from build123d import *

# Parameters (mm, degrees)
SKETCH1_W           = 120
SKETCH1_H           = 125
BOSS_EXTRUDE1_DEPTH = 70
SKETCH3_W           = 47
SKETCH3_H           = 9.5
CUT_EXTRUDE1_DEPTH  = 47
SKETCH4_W           = 43
SKETCH4_H           = 15
CUT_EXTRUDE2_DEPTH  = 47
CUT_REVOLVE1_ANGLE  = 120
SKETCH9_W           = 20
SKETCH9_H           = 47
CUT_EXTRUDE3_DEPTH  = 3
SKETCH10_W          = 20
SKETCH10_H          = 1.6
CUT_EXTRUDE4_DEPTH  = 3.5
CUT_EXTRUDE5_DEPTH  = 1
SKETCH13_W          = 71.5
SKETCH13_H          = 22.8
CUT_EXTRUDE6_DEPTH  = 5
SKETCH14_R          = 5
CUT_EXTRUDE7_DEPTH  = 10
SKETCH15_R          = 8
CUT_EXTRUDE8_DEPTH  = 1
SKETCH16_W          = 70
SKETCH16_H          = 18
CUT_EXTRUDE9_DEPTH  = 10
SKETCH17_W          = 70
SKETCH17_H          = 9
SKETCH18_W          = 70
SKETCH18_H          = 9
SKETCH19_W          = 60
SKETCH19_H          = 15
CUT_EXTRUDE10_DEPTH = 60
CUT_REVOLVE4_ANGLE  = 90
SKETCH21_W          = 120
SKETCH21_H          = 125
CUT_EXTRUDE11_DEPTH = 20
FILLET1_R           = 3
FILLET2_R           = 3
SKETCH22_W          = 11.5
SKETCH22_H          = 18.1
CUT_EXTRUDE12_DEPTH = 7


# Some blends are built 0.0001 mm under size
with BuildPart() as part:
    # Sketch1 → Boss-Extrude1 (new body)
    with BuildSketch(Plane(origin=(0, 0, 0), x_dir=(1, 0, 0), z_dir=(0, 1, 0))):
        with Locations((60, 62.5)):
            Rectangle(SKETCH1_W, SKETCH1_H)
    extrude(amount=BOSS_EXTRUDE1_DEPTH)

    # Sketch3 → Cut-Extrude1 (cut)
    with BuildSketch(Plane.XY):
        with Locations((26.5, 50.25)):
            Rectangle(SKETCH3_W, SKETCH3_H)
    extrude(amount=-CUT_EXTRUDE1_DEPTH, mode=Mode.SUBTRACT)

    # Sketch4 → Cut-Extrude2 (cut)
    with BuildSketch(Plane.XY):
        with Locations((26.5, 62.5)):
            Rectangle(SKETCH4_W, SKETCH4_H)
    extrude(amount=-CUT_EXTRUDE2_DEPTH, mode=Mode.SUBTRACT)

    # Cut-Sweep1: sweep along a path in Sketch5
    with BuildLine(Plane.XY) as cut_sweep1_path:
        Line((9, 45.5), (9, 33))
        ThreePointArc((9, 33), (10.464466094, 29.464466094), (14, 28))
        Line((14, 28), (39, 28))
        ThreePointArc((39, 28), (42.535533906, 29.464466094), (44, 33))
        Line((44, 33), (44, 45.5))
    # Sketch6 → Cut-Sweep1 (sweep, cut)
    with BuildSketch(Plane(origin=(0, 45.5, 0), x_dir=(1, 0, 0), z_dir=(0, 1, 0))):
        with BuildLine():
            Line((7, 0), (7, 2))
            ThreePointArc((7, 2), (9, 4), (11, 2))
            Line((11, 2), (11, 0))
            Line((11, 0), (7, 0))
        make_face()
    sweep(path=cut_sweep1_path.line, mode=Mode.SUBTRACT)

    # Sketch7 → Cut-Revolve1 (revolve, cut)
    with BuildSketch(Plane.XY):
        with BuildLine():
            Line((19.5, 30), (33.5, 30))
            ThreePointArc((33.5, 30), (26.5, 37), (19.5, 30))
        make_face()
    revolve(axis=Axis((19.5, 30, 0), (-1, 0, 0)), revolution_arc=CUT_REVOLVE1_ANGLE, mode=Mode.SUBTRACT)

    # Sketch9 → Cut-Extrude3 (cut)
    with BuildSketch(Plane(origin=(0, 45.5, 0), x_dir=(1, 0, 0), z_dir=(0, 1, 0))):
        with Locations((26.5, 23.5)):
            Rectangle(SKETCH9_W, SKETCH9_H)
    extrude(amount=-CUT_EXTRUDE3_DEPTH, mode=Mode.SUBTRACT)

    # Sketch10 → Cut-Extrude4 (cut)
    with BuildSketch(Plane.XY.offset(-47)):
        with Locations((26.5, 47.5)):
            Rectangle(SKETCH10_W, SKETCH10_H)
    extrude(amount=-CUT_EXTRUDE4_DEPTH, mode=Mode.SUBTRACT)

    # Sketch11 → Cut-Extrude5 (cut)
    with BuildSketch(Plane(origin=(0, 70, 0), x_dir=(1, 0, 0), z_dir=(0, 1, 0))):
        with BuildLine():
            Line((54.58, 81.89), (113.38, 81.89))
            ThreePointArc((113.38, 81.89), (116.972102448, 80.402102448), (118.46, 76.81))
            Line((118.46, 76.81), (118.46, 10.08))
            ThreePointArc((118.46, 10.08), (116.972102448, 6.487897552), (113.38, 5))
            Line((113.38, 5), (54.58, 5))
            ThreePointArc((54.58, 5), (50.987897552, 6.487897552), (49.5, 10.08))
            Line((49.5, 10.08), (49.5, 76.81))
            ThreePointArc((49.5, 76.81), (50.987897552, 80.402102448), (54.58, 81.89))
        make_face()
    extrude(amount=-CUT_EXTRUDE5_DEPTH, mode=Mode.SUBTRACT)

    # Sketch13 → Cut-Extrude6 (cut)
    with BuildSketch(Plane(origin=(0, 70, 0), x_dir=(1, 0, 0), z_dir=(0, 1, 0))):
        with Locations((64.25, 101.6)):
            Rectangle(SKETCH13_W, SKETCH13_H)
    extrude(amount=-CUT_EXTRUDE6_DEPTH, mode=Mode.SUBTRACT)

    # Sketch14 → Cut-Extrude7 (cut)
    with BuildSketch(Plane(origin=(0, 70, 0), x_dir=(1, 0, 0), z_dir=(0, 1, 0))):
        with Locations(Location((25, 67, 0), (0, 0, 270))):
            Circle(SKETCH14_R)
    extrude(amount=-CUT_EXTRUDE7_DEPTH, mode=Mode.SUBTRACT)

    # Sketch15 → Cut-Extrude8 (cut)
    with BuildSketch(Plane(origin=(0, 70, 0), x_dir=(1, 0, 0), z_dir=(0, 1, 0))):
        with Locations(Location((25, 67, 0), (0, 0, 270))):
            Circle(SKETCH15_R)
    extrude(amount=-CUT_EXTRUDE8_DEPTH, mode=Mode.SUBTRACT)

    # Sketch16 → Cut-Extrude9 (cut)
    with BuildSketch(Plane(origin=(120, 0, 0), x_dir=(0, 0, -1), z_dir=(1, 0, 0))):
        with Locations((80, 56)):
            Rectangle(SKETCH16_W, SKETCH16_H)
        with Locations((80, 36)):
            Rectangle(SKETCH16_W, SKETCH16_H)
    extrude(amount=-CUT_EXTRUDE9_DEPTH, mode=Mode.SUBTRACT)

    # Sketch17 → Cut-Revolve2 (revolve, cut)
    with BuildSketch(Plane(origin=(110, 0, 0), x_dir=(0, 0, -1), z_dir=(1, 0, 0))):
        with Locations((80, 60.5)):
            Rectangle(SKETCH17_W, SKETCH17_H)
    revolve(axis=Axis((110, 56, -45), (0, 0, -1)), mode=Mode.SUBTRACT)

    # Sketch18 → Cut-Revolve3 (revolve, cut)
    with BuildSketch(Plane(origin=(110, 0, 0), x_dir=(0, 0, -1), z_dir=(1, 0, 0))):
        with Locations((80, 40.5)):
            Rectangle(SKETCH18_W, SKETCH18_H)
    revolve(axis=Axis((110, 36, -45), (0, 0, -1)), mode=Mode.SUBTRACT)

    # Sketch19 → Cut-Extrude10 (cut)
    with BuildSketch(Plane.ZY):
        with Locations((-85, 37.5)):
            Rectangle(SKETCH19_W, SKETCH19_H)
    extrude(amount=-CUT_EXTRUDE10_DEPTH, mode=Mode.SUBTRACT)

    # Sketch20 → Cut-Revolve4 (revolve, cut)
    with BuildSketch(Plane.ZY):
        with BuildLine():
            Line((-95, 45), (-75, 45))
            ThreePointArc((-75, 45), (-85, 55), (-95, 45))
        make_face()
    revolve(axis=Axis((0, 45, -95), (0, 0, -1)), revolution_arc=CUT_REVOLVE4_ANGLE, mode=Mode.SUBTRACT)

    # Sketch21 → Cut-Extrude11 (cut)
    with BuildSketch(Plane.XZ):
        with Locations((60, -62.5)):
            Rectangle(SKETCH21_W, SKETCH21_H)
    extrude(amount=-CUT_EXTRUDE11_DEPTH, mode=Mode.SUBTRACT)

    # Fillet1
    fillet1_edges = [part.edges().sort_by_distance(p)[0] for p in [
        (60, 20, 0),
        (120, 20, -62.5),
        (60, 20, -125),
        (0, 20, -62.5),
        (0, 45, -125),
        (120, 45, -125),
        (120, 45, 0),
        (0, 45, 0),
    ]]
    fillet(fillet1_edges, radius=FILLET1_R - 0.0001)  # a hair under: the kernel refuses the full size

    # Fillet2
    # the kernel refuses this fillet: 3 mm, written as the material it takes off along each edge
    with BuildSketch(Plane(origin=(40.500249996, 70, 0), x_dir=(0, -0.9999999994444074, 3.3334444463032727e-05), z_dir=(1, 0, 0))) as fillet2_piece_1:
        with BuildLine():
            CenterArc((2.999799998, 2.999999998), FILLET2_R, 180.001909923, 90)
            Line((-0.0002, 2.999899995), (-0.0602, 2.999897995))
            ThreePointArc((-0.0602, 2.999897995), (-0.06005, 1.499947999), (-0.06, -2e-06))
            Line((-0.06, -2e-06), (2e-06, -0.06))
            ThreePointArc((2e-06, -0.06), (1.499951999, -0.05995), (2.999902002, -0.06))
            Line((2.999902002, -0.06), (2.999900002, 0))
        make_face()
    extrude(amount=76.499850004, mode=Mode.SUBTRACT)
    with BuildSketch(Plane(origin=(117.0001, 70, -2.9999), x_dir=(0, 0, 1), z_dir=(-1, 0, 0))) as fillet2_piece_2:
        with BuildLine():
            CenterArc((0, -2.9999), FILLET2_R, 0, 90)
            Line((3, -2.9999), (3.06, -2.9999))
            ThreePointArc((3.06, -2.9999), (3.0599, -1.49995), (3.0599, 0))
            Line((3.0599, 0), (2.9999, 0.06))
            ThreePointArc((2.9999, 0.06), (1.49995, 0.06), (0, 0.0601))
            Line((0, 0.0601), (0, 0.0001))
        make_face()
    revolve(axis=Axis((117.0001, 70, -2.9999), (0, 1, 0)), revolution_arc=90, mode=Mode.SUBTRACT)
    with BuildSketch(Plane(origin=(120, 70, -2.9999), x_dir=(-0.9999999994444074, 3.333444446406897e-05, 0), z_dir=(0, 0, -1)), Plane(origin=(0, 70, -122.0001), x_dir=(0.9999999994444074, 3.333444446406897e-05, 0), z_dir=(0, 0, 1))) as fillet2_piece_3:
        with BuildLine():
            CenterArc((2.999799998, -2.999999998), FILLET2_R, 89.998090077, 90)
            Line((-0.0002, -2.999899995), (-0.0602, -2.999897995))
            ThreePointArc((-0.0602, -2.999897995), (-0.06005, -1.499947999), (-0.06, 2e-06))
            Line((-0.06, 2e-06), (2e-06, 0.06))
            ThreePointArc((2e-06, 0.06), (1.499951999, 0.05995), (2.999902002, 0.06))
            Line((2.999902002, 0.06), (2.999900002, 0))
        make_face()
    extrude(amount=119.0002, mode=Mode.SUBTRACT)
    with BuildSketch(Plane(origin=(117.0001, 70, -122.0001), x_dir=(1, 0, 0), z_dir=(0, 0, 1))) as fillet2_piece_4:
        with BuildLine():
            CenterArc((0, -2.9999), FILLET2_R, 0, 90)
            Line((3, -2.9999), (3.06, -2.9999))
            ThreePointArc((3.06, -2.9999), (3.0599, -1.49995), (3.0599, 0))
            Line((3.0599, 0), (2.9999, 0.06))
            ThreePointArc((2.9999, 0.06), (1.49995, 0.06), (0, 0.0601))
            Line((0, 0.0601), (0, 0.0001))
        make_face()
    revolve(axis=Axis((117.0001, 70, -122.0001), (0, 1, 0)), revolution_arc=90, mode=Mode.SUBTRACT)
    with BuildSketch(Plane(origin=(117.0001, 70, -125), x_dir=(0, 3.333444446406897e-05, 0.9999999994444074), z_dir=(-1, 0, 0))) as fillet2_piece_5:
        with BuildLine():
            CenterArc((2.999799998, -2.999999998), FILLET2_R, 89.998090077, 90)
            Line((-0.0002, -2.999899995), (-0.0602, -2.999897995))
            ThreePointArc((-0.0602, -2.999897995), (-0.06005, -1.499947999), (-0.06, 2e-06))
            Line((-0.06, 2e-06), (2e-06, 0.06))
            ThreePointArc((2e-06, 0.06), (1.499951999, 0.05995), (2.999902002, 0.06))
            Line((2.999902002, 0.06), (2.999900002, 0))
        make_face()
    extrude(amount=114.0002, mode=Mode.SUBTRACT)
    with BuildSketch(Plane(origin=(2.9999, 70, -122.0001), x_dir=(-1, 0, 0), z_dir=(0, 0, 1))) as fillet2_piece_6:
        with BuildLine():
            CenterArc((0, 2.9999), FILLET2_R, 270, 90)
            Line((3, 2.9999), (3.06, 2.9999))
            ThreePointArc((3.06, 2.9999), (3.0599, 1.49995), (3.0599, 0))
            Line((3.0599, 0), (2.9999, -0.06))
            ThreePointArc((2.9999, -0.06), (1.49995, -0.06), (0, -0.0601))
            Line((0, -0.0601), (0, -0.0001))
        make_face()
    revolve(axis=Axis((2.9999, 70, -122.0001), (0, -1, 0)), revolution_arc=90, mode=Mode.SUBTRACT)
    with BuildSketch(Plane(origin=(2.9999, 70, 0), x_dir=(0, -0.9999999994444074, 3.3334444463032727e-05), z_dir=(1, 0, 0))) as fillet2_piece_7:
        with BuildLine():
            CenterArc((2.999799998, 2.999999998), FILLET2_R, 180.001909923, 90)
            Line((-0.0002, 2.999899995), (-0.0602, 2.999897995))
            ThreePointArc((-0.0602, 2.999897995), (-0.06005, 1.499947999), (-0.06, -2e-06))
            Line((-0.06, -2e-06), (2e-06, -0.06))
            ThreePointArc((2e-06, -0.06), (1.499951999, -0.05995), (2.999902002, -0.06))
            Line((2.999902002, -0.06), (2.999900002, 0))
        make_face()
    extrude(amount=9.499850004, mode=Mode.SUBTRACT)
    with BuildSketch(Plane(origin=(2.9999, 70, -2.9999), x_dir=(0, 0, 1), z_dir=(1, 0, 0))) as fillet2_piece_8:
        with BuildLine():
            CenterArc((0, 2.9999), FILLET2_R, 270, 90)
            Line((3, 2.9999), (3.06, 2.9999))
            ThreePointArc((3.06, 2.9999), (3.0599, 1.49995), (3.0599, 0))
            Line((3.0599, 0), (2.9999, -0.06))
            ThreePointArc((2.9999, -0.06), (1.49995, -0.06), (0, -0.0601))
            Line((0, -0.0601), (0, -0.0001))
        make_face()
    revolve(axis=Axis((2.9999, 70, -2.9999), (0, -1, 0)), revolution_arc=90, mode=Mode.SUBTRACT)

    # Sketch22 → Cut-Extrude12 (cut)
    with BuildSketch(Plane(origin=(120, 0, 0), x_dir=(0, 0, -1), z_dir=(1, 0, 0))):
        with Locations((21.75, 47.95)):
            Rectangle(SKETCH22_W, SKETCH22_H)
    extrude(amount=-CUT_EXTRUDE12_DEPTH, mode=Mode.SUBTRACT)


solid = part.part
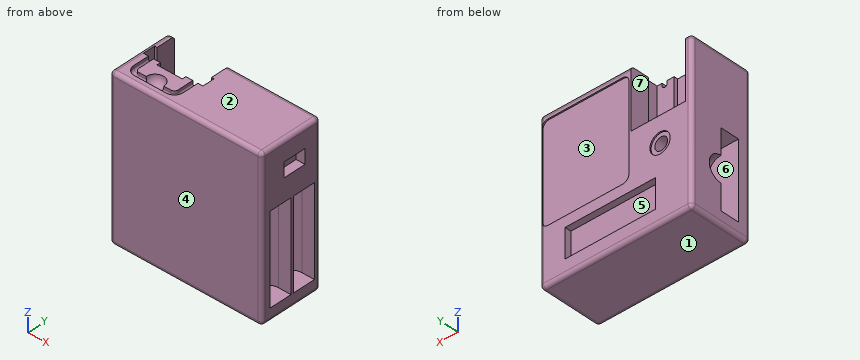
Read the model definition and answer for the solid it produces. Units are mm, in the model's axes. Face numbers are marked on the shaded views. A direction names the side the tool comes from. Coordinates: 2 decimals unless noted, no trailing zeros. Order: outer loops, then holes, each group sorted by start corner. A loop starts at its lowest first (then second) coordinate and runs counter-clockwise, first axis right, second up. Notation, with made-up numbers: (-2, 60) - (56, 60) arc R16 ccw to (56, 70) - close; hole circle Ø3 at (37, 6.5). An arc over 180 degrees is marked (long way). Use one line per item in the form item = value.
(1) Which of the six approach directions +Z, -Z, +X, -X, +Y, -Y give full straight-line access (tool end or side, diameter ignored) to the marked faces 5, 6 and 7?
Computed values:
face_5 = +Y
face_6 = -X
face_7 = +Z, +Y
(2) For a pull along Z with two mould halves and no side action, classify the marked faces 1, 2, 3 and 4 as pulls with the +Z half, pulls with the -Z half, needs draft (parallel to the pull), parting line crosses it, or undercut.
Computed values:
face_1 = pulls with the -Z half
face_2 = pulls with the +Z half
face_3 = undercut
face_4 = needs draft
(3) Section A-A, the plane x = 72.5 is taken. Give the vertices of the cut face in (y, z), then the cut area to 3 significant figures.
Computed values:
outline = (20, -122) arc R3 ccw to (23, -125) - (67.02, -125) arc R3 ccw to (70, -122.02) - (70, -113) - (65, -113) - (65, -90.2) - (70, -90.2) - (70, -81.89) - (69, -81.89) - (69, -5) - (70, -5) - (70, -2.98) arc R3 ccw to (67.02, 0) - (23, 0) arc R3 ccw to (20, -3) - close
area = 6,050 mm²
(4) Section D-D, the plane y = 58.5 is taken. Give the vertices of the cut face in (x, z).
Computed values:
outline = (0, -122) arc R3 ccw to (3, -125) - (117, -125) arc R3 ccw to (120, -122) - (120, -115) - (101.35, -115) - (101.35, -45) - (120, -45) - (120, -3) arc R3 ccw to (117, 0) - (48, 0) - (48, -47) - (5, -47) - (5, 0) - (3, 0) arc R3 ccw to (0, -3) - close
(5) Straight lines are drawn through the part: L1, parallel to Y at x = 7, z = -100; L2, parallel to X at y = 62.5, z = -32; L3, parallel to Z at x = 35, y = 34. For each, find the intervals that lie inside material, in ascending order.
Computed values:
L1 = 20 to 30, 45 to 70
L2 = 0 to 5, 48 to 120
L3 = -125 to -115, -55 to 0
(6) Given pin 1 Ø1.6 at (y, z) = (38.5, -1) entering from -X; pin 2 Ø1.5 at (x, z) = (100.5, -67) entering from +Y; pin 3 Ø2 at (y, z) = (42, -0.5) entering from -X, each flat-ended and moving along its own axis, determine where each tip first touches the part or whether it passes through.
Computed values:
pin_1 = 0.25
pin_2 = 69
pin_3 = 0.4
